The listing builds one solid part. Answer for the finished solid, in the listing's coordinates (mm). Face numbers are marked on the shaded views. A direction names the side the tool comes from. Round coordinates to 2 decimals unless told otherwise and drop trailing zeros. Write each loop counter-clockwise with the first axis right and the second up, starting at its lowest first coordinate (ties: lowest second). Pieces come first, ordered by that corner, then holes.
from build123d import *

# Parameters (mm, degrees)
BOSS_EXTRUDE1_DEPTH = 1.5875
SKETCH2_W           = 26.5
SKETCH2_H           = 127
BOSS_EXTRUDE2_DEPTH = 1.5875


with BuildPart() as part:
    # Sketch1 → Boss-Extrude1 (new body)
    with BuildSketch(Plane.XY):
        Polygon((-26.5, 120), (0, 120), (0, 0), (-26.5, 0), (-26.5, 3.5), (-11.5, 20.5), (-5.4, 20.5), (-5.4, 99.5), (-11.5, 99.5), (-26.5, 116.5), align=None)
        with BuildLine():
            ThreePointArc((-14.15, 112.5), (-12.5, 110.85), (-10.85, 112.5))
            ThreePointArc((-10.85, 112.5), (-12.5, 114.15), (-14.15, 112.5))
        make_face(mode=Mode.SUBTRACT)
        with BuildLine():
            ThreePointArc((-14.15, 7.5), (-12.5, 5.85), (-10.85, 7.5))
            ThreePointArc((-10.85, 7.5), (-12.5, 9.15), (-14.15, 7.5))
        make_face(mode=Mode.SUBTRACT)
    extrude(amount=BOSS_EXTRUDE1_DEPTH)

    # Sketch2 → Boss-Extrude2 (add)
    with BuildSketch(Plane(origin=(0, 0, 0), x_dir=(1, 0, 0), z_dir=(0, 1, 0))):
        with Locations((-13.25, 61.9125)):
            Rectangle(SKETCH2_W, SKETCH2_H)
    extrude(amount=-BOSS_EXTRUDE2_DEPTH)


solid = part.part
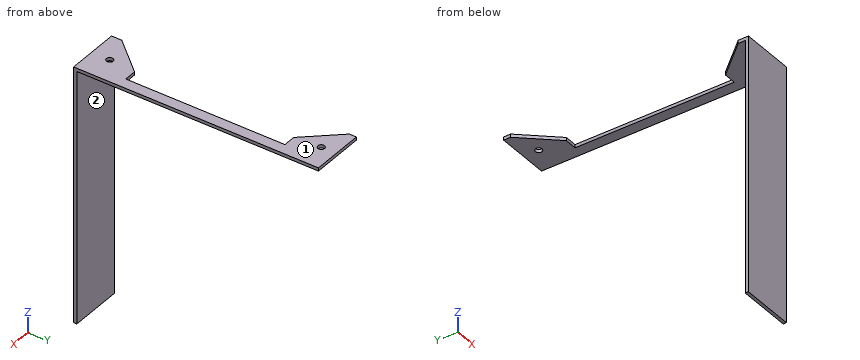
1. A tool of negligible diameter and unlimited length cuts with its end or side. For the marked faces 1 and 2, from which of +Z, -Z, +X, -X, +Y, -Y can it reach the whole face along a straight path? Write none if from no direction.
Geometry says:
face 1: +Z, +X, -X, +Y, -Y
face 2: -Z, +X, -X, +Y
2. Section A-A on x = -8.75 is taken. Determine the outline of the cut face in (y, z).
Geometry says:
outline: (-1.59, -125.41) - (0, -125.41) - (0, 0) - (20.5, 0) - (20.5, 1.59) - (-1.59, 1.59) - close; (99.5, 0) - (120, 0) - (120, 1.59) - (99.5, 1.59) - close
3. Straight lines are drawn through the part: line 1 along Y through (x, z) = (-12.5, 0.7); line 2 along Y through (x, z) = (-2.5, -65.5); line 3 along X through (y, z) = (7, 1). For each, find the intervals that lie inside material, in ascending order.
Geometry says:
line 1: y = -1.59 to 5.85, 9.15 to 19.37, 100.63 to 110.85, 114.15 to 120
line 2: y = -1.59 to 0
line 3: x = -23.41 to -14.07, -10.93 to 0
4. Section D-D on y = 26 is taken. Determine the outline of the cut face in (x, z), plus the area to 3 significant figures.
Geometry says:
outline: (-5.4, 0) - (0, 0) - (0, 1.59) - (-5.4, 1.59) - close
area: 8.57 mm2
5. Given pin 1 (5 mm diameter, centred on x = -19.5, z = -57, fed in from +Y); pin 2 (0.8 mm diameter, centred on y = 57, z = 1, fed in from -X), each flat-ended and moving along its own axis, determine where each tip first touches the part or whether it passes through.
Geometry says:
pin 1: stops at y = 0
pin 2: stops at x = -5.4
6. Section B-B on y = 112.5 is taken. Determine the outline of the cut face in (x, z), plus the area to 3 significant figures.
Geometry says:
outline: (-22.97, 0) - (-14.15, 0) - (-14.15, 1.59) - (-22.97, 1.59) - close; (-10.85, 0) - (0, 0) - (0, 1.59) - (-10.85, 1.59) - close
area: 31.2 mm2
7. Section C-C on x = -20.5 is taken. Determine the outline of the cut face in (y, z), plus the area to 3 significant figures.
Geometry says:
outline: (-1.59, -125.41) - (0, -125.41) - (0, 0) - (10.3, 0) - (10.3, 1.59) - (-1.59, 1.59) - close; (109.7, 0) - (120, 0) - (120, 1.59) - (109.7, 1.59) - close
area: 234 mm2
